Autodesk Inventor part; units mm, degrees
ref_plane "YZ Plane" through (0, 0, 0) normal (1, 0, 0) x (0, 1, 0)
ref_plane "XZ Plane" through (0, 0, 0) normal (0, 1, 0) x (-1, 0, 0)
ref_plane "XY Plane" through (0, 0, 0) normal (0, 0, 1) x (1, 0, 0)
sketch "Náčrt1" plane through (0, 0, 0) normal (0, 0, 1) x (1, 0, 0)
  line L0 (-5, 8) -> (-5, 0)
  line L1 (-5, 0) -> (5, 0)
  line L2 (5, 0) -> (5, 8)
  line L3 (5, 8) -> (3.5, 8)
  line L4 (3.5, 8) -> (3.5, 1.5)
  line L5 (3.5, 1.5) -> (-3.5, 1.5)
  line L6 (-3.5, 1.5) -> (-3.5, 8)
  line L7 (-3.5, 8) -> (-5, 8)
  line L8 (-7, 0) -> (7, 0)
  line L9 (0, 9.6) -> (0, -1.6)
  point P0 (0, 0)
  dimension "d0" = 8
  dimension "d1" = 10
  dimension "d2" = 1.5
  dimension "d3" = 1.5
  dimension "d4" = 1.5
extrude "Vysunutí1" add sketch "Náčrt1" along normal mid plane 30
sketch "Náčrt2" plane through (5, 0, 15) normal (1, 0, 0) x (0, 0, -1)
  line L0 (30, 8) -> (30, 0)
  line L1 (0, 0) -> (0, 8)
  line L2 (30, 8) -> (0, 8)
  point P0 (15, 0)
  point P1 (5, 4.5)
  point P2 (25, 4.5)
  dimension "d7" = 5
  dimension "d8" = 5
  dimension "d9" = 3.5
  dimension "d10" = 3.5
hole "Díra1" at (5, 4.5, 10) at (5, 4.5, -10) direction (-1, 0, 0) diameter 2.459 end through all counterbore diameter 3.2 counterbore depth 2
sketch "Náčrt3" plane through (-3.5, 1.5, 15) normal (0, 1, 0) x (1, 0, 0)
  line L0 (0, 30) -> (0, 0)
  point P0 (3.5, 15)
  point P1 (3.5, 10)
  point P2 (3.5, 20)
  dimension "d18" = 10
  dimension "d19" = 5
  dimension "d20" = 3.5
  dimension "d21" = 3.5
hole "Díra2" at (0, 1.5, 5) at (0, 1.5, -5) direction (0, -1, 0) diameter 2.459 end through all
properties part number "y_belt_anchor" material "Hliník 6061"
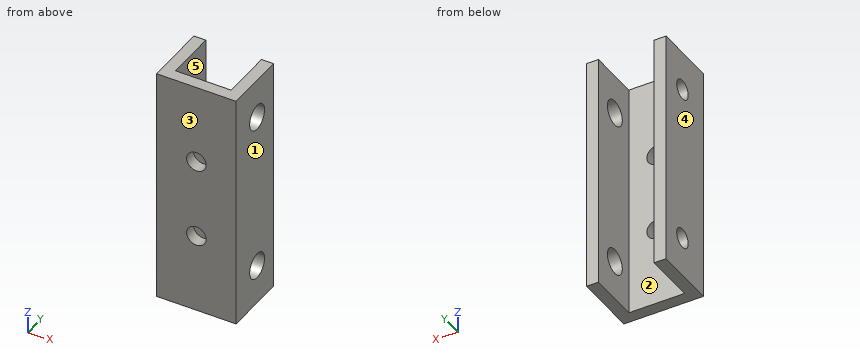
CAD build for the part. Positions are in the model's coordinates, mm. Face numbers are marked on the shaded views. A direction names the side the tool comes from. Round coordinates to 2 decimals unless told otherwise and drop trailing zeros. Loops run counter-clockwise (first coordinate to the right, second up) from the corner with the lowest first, then second, coordinate; pieces in that order, holes last. Notation, with made-up numbers: M 13.25,-4 L 65.25,-4 A11 ccw 65.25,6 Z; hole C 18,18.25 d7. An arc over 180 degrees is marked long. Return JSON: item names as keys, results as strings. Group by question number.
(1) Saw through at C-C, the plane x = 0. List the corners of the cut face in (y, z), and give its area (3 significant figures).
(2) Saw through at A-A, the plane z = -5. List the corners of the cut face in (x, y), and give its area (3 significant figures).
(3) Mould opens along X. For the marked faces 1, 2 and 3 say: +X half, -X half, draft (parallel to the pull), parting line (faces both ways), or undercut.
(4) Drop flat-ended pins along their axis: P1, Ø2, axis at x = 0.5, y = 4, coming from the -Z side; P2, Ø3, axis at y = 4.5, z = -10, coming from the +X side; P3, Ø4, axis at y = 4.5, z = 10, coming from the -X side; P4, Ø2, axis at x = 1, z = 2.5, coming from the +Y side. Give the stop position or say it passes through.
(5) Saw through at B-B, the plane y = 4.5. List the corners of the cut face in (x, z), and give its area (3 significant figures).
(6) Tool access for the marked faces 4 and 5: list every direction of +Z, -Z, +X, -X, +Y, -Y with a clear straight run to the whole face (end or side of a thin tool).
(7) Wall check: probe 1 along Z at (x, y) = (0, 0.8); probe 2 along Z at (x, y) = (-4.45, 4.5); probe 3 along X at (y, z) = (5.25, -8). Give the ranges that are in metal, low to high. Write a range as [from, to].
(8) Saw through at D-D, the plane y = 7.5. List the corners of the cut face in (x, z).
Answer list:
{
 "1": {"outline": "M 0,-15 L 1.5,-15 L 1.5,-6.23 L 0,-6.23 Z; M 0,-3.77 L 1.5,-3.77 L 1.5,3.77 L 0,3.77 Z; M 0,6.23 L 1.5,6.23 L 1.5,15 L 0,15 Z", "area": "37.6 mm2"},
 "2": {"outline": "M -5,0 L -1.23,0 L -1.23,1.5 L -3.5,1.5 L -3.5,8 L -5,8 Z; M 1.23,0 L 5,0 L 5,8 L 3.5,8 L 3.5,1.5 L 1.23,1.5 Z", "area": "30.8 mm2"},
 "3": {"face 1": "+X half", "face 2": "undercut", "face 3": "draft"},
 "4": {"P1": "through", "P2": "x = -3.5", "P3": "x = -5", "P4": "y = 1.5"},
 "5": {"outline": "M -5,-15 L -3.5,-15 L -3.5,-11.23 L -5,-11.23 Z; M -5,-8.77 L -3.5,-8.77 L -3.5,8.77 L -5,8.77 Z; M -5,11.23 L -3.5,11.23 L -3.5,15 L -5,15 Z; M 3.5,-15 L 5,-15 L 5,-11.6 L 3.5,-11.6 Z; M 3.5,-8.4 L 5,-8.4 L 5,8.4 L 3.5,8.4 Z; M 3.5,11.6 L 5,11.6 L 5,15 L 3.5,15 Z", "area": "73.0 mm2"},
 "6": {"face 4": "+Z, -Z, -X, +Y, -Y", "face 5": "+Z, -Z, +Y"},
 "7": {"probe 1": "[-15, -6.23], [-3.77, 3.77], [6.23, 15]", "probe 2": "[-15, -11.23], [-8.77, 8.77], [11.23, 15]", "probe 3": "[-5, -3.5], [3.5, 5]"},
 "8": {"outline": "M -5,-15 L -3.5,-15 L -3.5,15 L -5,15 Z; M 3.5,-15 L 5,-15 L 5,15 L 3.5,15 Z"}
}
